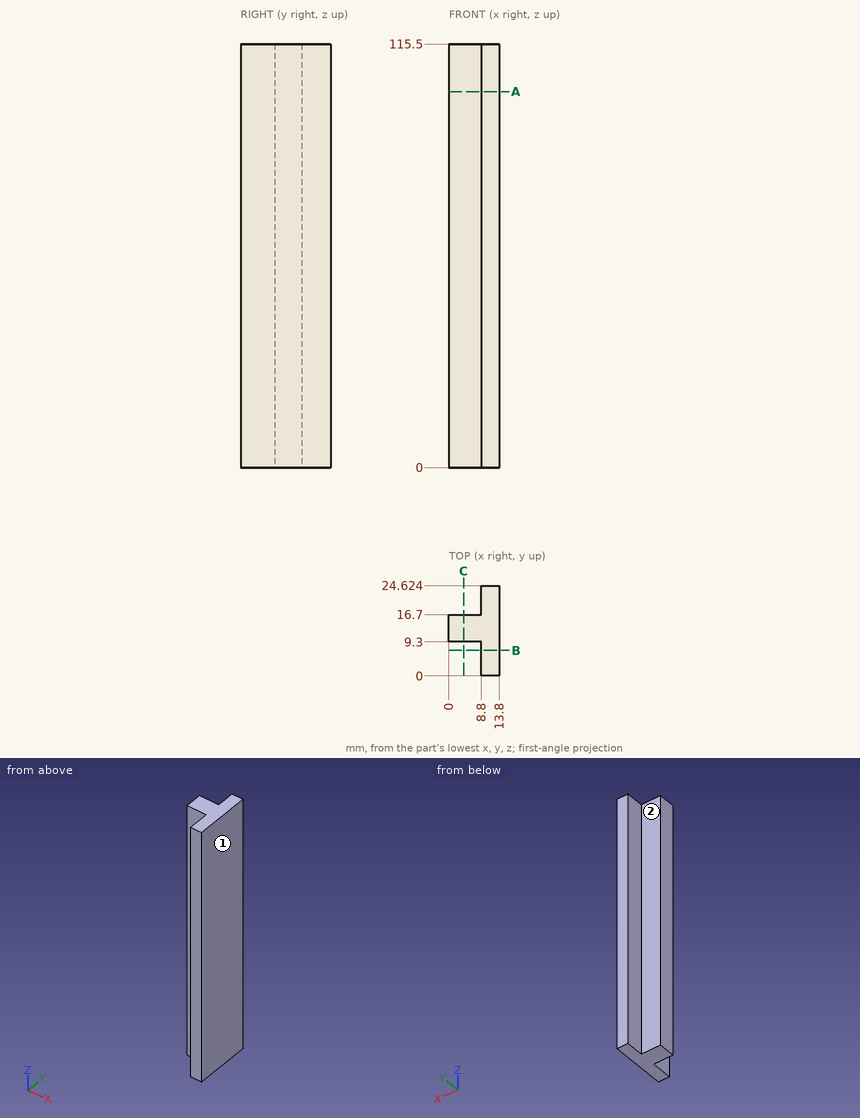
Input: dimensioned drawing with shaded views. Units: mm. Origin: part minimum x, y, z. A direction names the side the tool comes from. Round coordinates to 2 decimals unless told otherwise and drop trailing zeros. Loops run counter-clockwise (first coordinate to the right, second up) from the corner with the lowest first, then second, coordinate; pieces in that order, holes last.
1) Section query A-A on z = 102.5. Return the cut outline in (x, y), plus the area to 3 significant figures.
Ans:
outline: (0, 9.3) - (8.8, 9.3) - (8.8, 0) - (13.8, 0) - (13.8, 24.62) - (8.8, 24.62) - (8.8, 16.7) - (0, 16.7) - close
area: 188 mm2
2) Material intervals for line 1 (Y direction, x = 7.25, z = 14); line 2 (X direction, y = 6, z = 111.5), sorted ascending.
Ans:
line 1: y = 9.3 to 16.7
line 2: x = 8.8 to 13.8
3) Pin query (flat end, axial travel): pin 1 (1 mm diameter, centred on x = 5, z = 27.5, fed in from +Y); pin 2 (1.5 mm diameter, centred on x = 2.5, z = 74.5, fed in from -Y). Return the tip coordinate at first contact, or that it passes through.
Ans:
pin 1: stops at y = 16.7
pin 2: stops at y = 9.3
4) Set-up query: the marked faces 1 and 2. Return all of +Z, -Z, +X, -X, +Y, -Y with unobstructed straight access to the full face (end or side cutting, diameter ignored); none if empty.
Ans:
face 1: +Z, -Z, +X, +Y, -Y
face 2: +Z, -Z, -X, +Y
5) Section query C-C on x = 4. Return the cut outline in (y, z).
Ans:
outline: (9.3, 0) - (16.7, 0) - (16.7, 115.5) - (9.3, 115.5) - close
6) Section query B-B on y = 7. Return the cut outline in (x, z).
Ans:
outline: (8.8, 0) - (13.8, 0) - (13.8, 115.5) - (8.8, 115.5) - close
